from build123d import *

# Parameters (mm, degrees)
SKETCH1_W               = 50
SKETCH1_H               = 34.11
BOSS_EXTRUDE1_DEPTH     = 10
SKETCH3_W               = 41
SKETCH3_H               = 21
BOSS_EXTRUDE2_DEPTH     = 3
SKETCH2_W               = 3.5
SKETCH2_H               = 31
CUT_EXTRUDE1_DEPTH      = 4
CUT_EXTRUDE1_DEPTH_BACK = 7
SKETCH4_W               = 25
SKETCH4_H               = 21
BOSS_EXTRUDE3_DEPTH     = 20
SKETCH5_R               = 8.35
CUT_EXTRUDE2_DEPTH      = 30
SKETCH6_R               = 3.35
BOSS_EXTRUDE4_DEPTH     = 9.5
LPATTERN1_COUNT         = 3
LPATTERN1_PITCH         = 20.25
MIRROR1_COPY_1_SKETCH_R = 3.35
MIRROR1_COPY_1_DEPTH    = 9.5
MIRROR1_COPY_2_SKETCH_R = 3.35
MIRROR1_COPY_2_DEPTH    = 9.5
FILLET1_R               = 6
SKETCH7_W               = 23
SKETCH7_H               = 21
CUT_EXTRUDE3_DEPTH      = 0.5
FILLET2_R               = 6


with BuildPart() as part:
    # Sketch1 → Boss-Extrude1 (new body)
    with BuildSketch(Plane.XY):
        Rectangle(SKETCH1_W, SKETCH1_H)
    extrude(amount=BOSS_EXTRUDE1_DEPTH)

    # Sketch3 → Boss-Extrude2 (add)
    with BuildSketch(Plane(origin=(0, 0, 0), x_dir=(-1, 0, 0), z_dir=(0, 0, -1))):
        Rectangle(SKETCH3_W, SKETCH3_H)
    extrude(amount=BOSS_EXTRUDE2_DEPTH)

    # Sketch2 → Cut-Extrude1 (cut, two sides)
    with BuildSketch(Plane(origin=(0, 0, 0), x_dir=(-1, 0, 0), z_dir=(0, 0, -1))) as cut_extrude1_sk:
        with Locations((-14.25, 0)):
            Rectangle(SKETCH2_W, SKETCH2_H)
        with Locations((14.25, 0)):
            Rectangle(SKETCH2_W, SKETCH2_H)
    extrude(amount=CUT_EXTRUDE1_DEPTH, mode=Mode.SUBTRACT)
    extrude(cut_extrude1_sk.sketch, amount=-CUT_EXTRUDE1_DEPTH_BACK, mode=Mode.SUBTRACT)

    # Sketch4 → Boss-Extrude3 (add)
    with BuildSketch(Plane(origin=(0, 0, -3), x_dir=(-1, 0, 0), z_dir=(0, 0, -1))):
        Rectangle(SKETCH4_W, SKETCH4_H)
    extrude(amount=BOSS_EXTRUDE3_DEPTH)

    # Sketch5 → Cut-Extrude2 (cut)
    with BuildSketch(Plane(origin=(0, 0, -23), x_dir=(-1, 0, 0), z_dir=(0, 0, -1))):
        Circle(SKETCH5_R)
    extrude(amount=-CUT_EXTRUDE2_DEPTH, mode=Mode.SUBTRACT)

    # Sketch6 → Boss-Extrude4 (add)
    with BuildSketch(Plane(origin=(25, 0, 0), x_dir=(0, 0, -1), z_dir=(1, 0, 0))):
        with BuildLine():
            Line((-17, 27.1), (-7, 27.1))
            Line((-7, 27.1), (-2, 17.055))
            Line((-2, 17.055), (-10, 17.055))
            Line((-10, 17.055), (-10, 14.9))
            Line((-10, 14.9), (-17, 14.9))
            ThreePointArc((-17, 14.9), (-23.1, 21), (-17, 27.1))
        make_face()
        with Locations((-17, 21)):
            Circle(SKETCH6_R, mode=Mode.SUBTRACT)
    boss_extrude4 = extrude(amount=-BOSS_EXTRUDE4_DEPTH)

    # LPattern1: Boss-Extrude4 ×3
    with Locations(*[(-i * LPATTERN1_PITCH, 0, 0) for i in range(1, LPATTERN1_COUNT)]):
        add(boss_extrude4)

    # Mirror1: Boss-Extrude4 across plane
    add(boss_extrude4.mirror(Plane.ZX))

    # Mirror1 copy 1 sketch → Mirror1 copy 1 (add)
    with BuildSketch(Plane(origin=(4.75, 0, 0), x_dir=(0, 0, -1), z_dir=(1, 0, 0))):
        with BuildLine():
            Line((-17, -27.1), (-7, -27.1))
            Line((-7, -27.1), (-2, -17.055))
            Line((-2, -17.055), (-10, -17.055))
            Line((-10, -17.055), (-10, -14.9))
            Line((-10, -14.9), (-17, -14.9))
            ThreePointArc((-17, -14.9), (-23.1, -21), (-17, -27.1))
        make_face()
        with Locations((-17, -21)):
            Circle(MIRROR1_COPY_1_SKETCH_R, mode=Mode.SUBTRACT)
    extrude(amount=-MIRROR1_COPY_1_DEPTH)

    # Mirror1 copy 2 sketch → Mirror1 copy 2 (add)
    with BuildSketch(Plane(origin=(-15.5, 0, 0), x_dir=(0, 0, -1), z_dir=(1, 0, 0))):
        with BuildLine():
            Line((-17, -27.1), (-7, -27.1))
            Line((-7, -27.1), (-2, -17.055))
            Line((-2, -17.055), (-10, -17.055))
            Line((-10, -17.055), (-10, -14.9))
            Line((-10, -14.9), (-17, -14.9))
            ThreePointArc((-17, -14.9), (-23.1, -21), (-17, -27.1))
        make_face()
        with Locations((-17, -21)):
            Circle(MIRROR1_COPY_2_SKETCH_R, mode=Mode.SUBTRACT)
    extrude(amount=-MIRROR1_COPY_2_DEPTH)

    # Fillet1
    fillet1_edges = [part.edges().sort_by_distance(p)[0] for p in [
        (20.25, 27.1, 7),
        (20.25, 14.9, 10),
        (0, 27.1, 7),
        (0, 14.9, 10),
        (-20.25, 27.1, 7),
        (-20.25, 14.9, 10),
        (20.25, -14.9, 10),
        (20.25, -27.1, 7),
        (0, -14.9, 10),
        (0, -27.1, 7),
        (-20.25, -14.9, 10),
        (-20.25, -27.1, 7),
    ]]
    fillet(fillet1_edges, radius=FILLET1_R)

    # Sketch7 → Cut-Extrude3 (cut)
    with BuildSketch(Plane(origin=(12.5, 0, 0), x_dir=(0, 0, -1), z_dir=(1, 0, 0))):
        with Locations((11.5, 0)):
            Rectangle(SKETCH7_W, SKETCH7_H)
    cut_extrude3 = extrude(amount=-CUT_EXTRUDE3_DEPTH, mode=Mode.SUBTRACT)

    # Mirror2: Cut-Extrude3 across plane
    add(cut_extrude3.mirror(Plane(origin=(0, 0, 0), x_dir=(0, 0, 1), z_dir=(1, 0, 0))), mode=Mode.SUBTRACT)

    # Fillet2
    fillet2_edges = [part.edges().sort_by_distance(p)[0] for p in [
        (10.125, 17.055, 10),
        (-10.125, 17.055, 10),
        (10.125, -17.055, 10),
        (-10.125, -17.055, 10),
    ]]
    fillet(fillet2_edges, radius=FILLET2_R)


solid = part.part
Input: part model. Units: mm. Frame: model coordinates. A direction names the side the tool comes from. Give positions to 0.01 mm unless a question says otherwise; leave off trailing zeros. Loops run counter-clockwise (first coordinate to the right, second up) from the corner with the lowest first, then second, coordinate; pieces in that order, holes last. Notation, with made-up numbers: M -21,-2 L 38,-2 A9 cw 38,15 Z; hole C -27,-6.5 d11. An arc over 180 degrees is marked long. Use one line per item in the form item = value.
1. Section query D-D, the plane y = 0. Return the cut outline in (x, z), and give its area (3 significant figures).
Numbers:
outline = M -25,0 L -20.5,0 L -20.5,-3 L -16,-3 L -16,7 L -12.5,7 L -12.5,0 L -12,0 L -12,-23 L -8.35,-23 L -8.35,7 L 8.35,7 L 8.35,-23 L 12,-23 L 12,0 L 12.5,0 L 12.5,7 L 16,7 L 16,-3 L 20.5,-3 L 20.5,0 L 25,0 L 25,10 L -25,10 Z
area = 529 mm²
2. Reachability of faces 1 (the face through (-18, 10.5, -1)), 2 (the face through (10.2, -15.25, 8.29)), 3 (the face through (-0.3, 17.055, 1.5)), 4 (the face through (20.184, -13.096, 11.711)) from +Z, -Z, +X, -X, +Y, -Y: full face, straight path, thin tool, end or side. Return the list, or none.
Numbers:
face_1 = -Z, +X, -X, +Y
face_2 = +Z, -Y
face_3 = -Z, +Y
face_4 = +Z, +X, -X
3. Line query: L1, parallel to Y at x = -1.75, z = 17; L2, parallel to X at y = -13, z = 5.5; L3, parallel to Y at x = 2.5, z = 19. Output: solid intervals per line, ascending.
Numbers:
L1 = -27.1 to -24.35, -17.65 to -14.9, 14.9 to 17.65, 24.35 to 27.1
L2 = -25 to -16, -12.5 to 12.5, 16 to 25
L3 = -26.76 to -23.69, -18.31 to -15.24, 15.24 to 18.31, 23.69 to 26.76
4. Section query C-C, the plane y = 21. Return the cut outline in (x, z).
Numbers:
outline = M -25,3.96 L -15.5,3.96 L -15.5,13.65 L -25,13.65 Z; M -25,20.35 L -15.5,20.35 L -15.5,23.1 L -25,23.1 Z; M -4.75,3.96 L 4.75,3.96 L 4.75,13.65 L -4.75,13.65 Z; M -4.75,20.35 L 4.75,20.35 L 4.75,23.1 L -4.75,23.1 Z; M 15.5,3.96 L 25,3.96 L 25,13.65 L 15.5,13.65 Z; M 15.5,20.35 L 25,20.35 L 25,23.1 L 15.5,23.1 Z
5. Section query A-A, the plane x = -18. Return the cut outline in (y, z) (3 decimals), and give its area (3 significant figures).
Numbers:
outline = M -27.1,10.716 A6 ccw -23.774,5.344 L -17.055,2 L -17.055,0 L -10.5,0 L -10.5,-3 L 10.5,-3 L 10.5,0 L 17.055,0 L 17.055,2 L 23.774,5.344 A6 ccw 27.1,10.716 L 27.1,17 A6.1 ccw 14.9,17 L 14.9,16 A6 cw 8.9,10 L -8.9,10 A6 cw -14.9,16 L -14.9,17 A6.1 ccw -27.1,17 Z; hole C -21,17 d6.7; hole C 21,17 d6.7
area = 743 mm²
6. Section query B-B, the plane z = -12.5. Return the cut outline in (x, y).
Numbers:
outline = M -12,-10.5 L 12,-10.5 L 12,10.5 L -12,10.5 Z; hole C 0,0 d16.7
7. First-contact query: pin 1 (18.5 mm diameter, centred on x = 5, z = -12, fed in from -Y); pin 2 (3.5 mm diameter, centred on x = -19, z = -1.5, fed in from +Y) (3 decimals); pin 3 (24.5 mm diameter, centred on x = 7.5, y = -5.5, fed in from +Z); pin 4 (5.5 mm diameter, centred on y = 14, z = 14.5, fed in from -X). Flat tips, straight axial feed; report the tip coordinate or a pass-through.
Numbers:
pin_1 = -10.5
pin_2 = 17.055
pin_3 = 21.95
pin_4 = -25
8. Pull-direction query (X, two-part tool) for faces 5 (the face through (-14, 0, 7)), 6 (the face through (18, -10.5, -1)); classes: released by +X, released by -X, zero draft, split by the parting line, or undercut.
Numbers:
face_5 = undercut
face_6 = zero draft
